Geometry: final body of the model. Coordinates: model frame, mm. Face numbers are marked on the shaded views. A direction names the side the tool comes from. Give positions to 0.01 mm unless a question says otherwise; leave off trailing zeros. Order: outer loops, then holes, each group sorted by start corner. A loop starts at its lowest first (then second) coordinate and runs counter-clockwise, first axis right, second up. Notation, with made-up numbers: (51, 2.25) - (87, 2.25) arc R8 cw to (87, 6.25) - close; hole circle Ø11 at (88, -9). An arc over 180 degrees is marked (long way). Put each result on its own line as item: value. Start each with the question number.
1. Section A-A on y = 0.75. Return the cut outline in (x, z).
2. Section B-B on x = -12.7. Return the cut outline in (y, z), plus the area to 4 significant figures.
3. Ray query, line 1 along X through (y, z) = (5, 1.25); line 2 along Y through (x, z) = (12.7, 0.15); line 3 along X through (y, z) = (-4, 1.65). Return the intervals inside material, ascending. Write a range as from..to.
4. Section C-C on x = 21.5. Return the cut outline in (y, z).
5. Set-up query: the marked faces 1 and 2. Return all of +Z, -Z, +X, -X, +Y, -Y with unobstructed straight access to the full face (end or side cutting, diameter ignored); none if empty.
6. First-contact query: P1, Ø1.5, axis at y = 7.5, z = 1, coming from the +X side; P2, Ø0.8, axis at y = 4.5, z = 1, coming from the +X side; P3, Ø0.8, axis at x = 3.5, y = -10, coming from the -Z side. Flat tips, straight axial feed; report the tip coordinate or a pass-through.
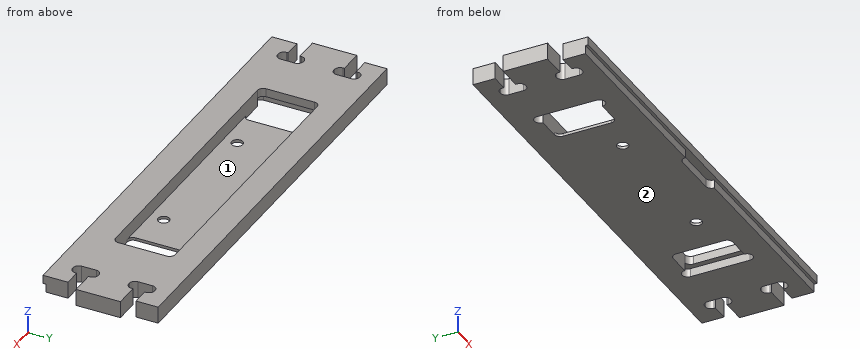
from build123d import *

# Parameters (mm, degrees)
SKETCH1_W                          = 1.3
SKETCH1_H                          = 7.9
BASE_SHAPE_DEPTH                   = 3
SKETCH4_W                          = 79
SKETCH4_H                          = 1.5
FLOOR_LIP_DEPTH                    = 0.5
NAIL_CUTOUT_DEPTH                  = 1.5
MILL_FILLETS_R                     = 1
LED_STRIP_POCKET_DEPTH             = 2.5
LED_STRIP_CUTS_REACH               = 2.5
SKETCH9_R                          = 1
LED_STRIP_CUT_FILLETS_R            = 1
LED_PCB_PADS_CLEARANCE_SLOTS_DEPTH = 1.5


with BuildPart() as part:
    # Sketch1 → Base shape (new body)
    with BuildSketch(Plane.XY):
        Polygon((39.5, 10), (-39.5, 10), (-39.5, 6.05), (-36.5, 6.05), (-36.5, 7.3), (-34.3, 7.3), (-34.3, 2.7), (-36.5, 2.7), (-36.5, 3.95), (-39.5, 3.95), (-39.5, -3.95), (-36.5, -3.95), (-36.5, -2.7), (-34.3, -2.7), (-34.3, -7.3), (-36.5, -7.3), (-36.5, -6.05), (-39.5, -6.05), (-39.5, -10), (39.5, -10), (39.5, -6.05), (36.5, -6.05), (36.5, -7.3), (34.3, -7.3), (34.3, -2.7), (36.5, -2.7), (36.5, -3.95), (39.5, -3.95), (39.5, 3.95), (36.5, 3.95), (36.5, 2.7), (34.3, 2.7), (34.3, 7.3), (36.5, 7.3), (36.5, 6.05), (39.5, 6.05), align=None)
        with Locations((-40.15, 0)):
            Rectangle(SKETCH1_W, SKETCH1_H)
        with Locations((40.15, 0)):
            Rectangle(SKETCH1_W, SKETCH1_H)
    extrude(amount=BASE_SHAPE_DEPTH)

    # Sketch4 → Floor lip (add)
    with BuildSketch(Plane.XZ.offset(10)):
        with Locations((0, 2.25)):
            Rectangle(SKETCH4_W, SKETCH4_H)
    extrude(amount=FLOOR_LIP_DEPTH)

    # Sketch6 → Nail cutout (cut)
    with BuildSketch(Plane(origin=(0, 0, 0), x_dir=(-1, 0, 0), z_dir=(0, 0, -1))):
        with BuildLine():
            Line((-4, -9), (4, -9))
            ThreePointArc((4, -9), (5, -10), (4, -11))
            Line((4, -11), (-4, -11))
            ThreePointArc((-4, -11), (-5, -10), (-4, -9))
        make_face()
    extrude(amount=-NAIL_CUTOUT_DEPTH, mode=Mode.SUBTRACT)

    # Mill fillets
    mill_fillets_edges = [part.edges().sort_by_distance(p)[0] for p in [
        (36.5, -2.7, 1.5),
        (34.3, -2.7, 1.5),
        (34.3, -7.3, 1.5),
        (36.5, -7.3, 1.5),
        (-36.5, -7.3, 1.5),
        (-34.3, -7.3, 1.5),
        (-34.3, -2.7, 1.5),
        (-36.5, -2.7, 1.5),
        (-36.5, 2.7, 1.5),
        (-34.3, 2.7, 1.5),
        (-34.3, 7.3, 1.5),
        (-36.5, 7.3, 1.5),
        (36.5, 7.3, 1.5),
        (34.3, 7.3, 1.5),
        (34.3, 2.7, 1.5),
        (36.5, 2.7, 1.5),
    ]]
    fillet(mill_fillets_edges, radius=MILL_FILLETS_R)

    # Sketch8 → Led strip pocket (cut)
    with BuildSketch(Plane.XY.offset(3)):
        with BuildLine():
            Line((-24.5, 5.3), (24.5, 5.3))
            ThreePointArc((24.5, 5.3), (25.207106781, 5.007106781), (25.5, 4.3))
            Line((25.5, 4.3), (25.5, -4.3))
            ThreePointArc((25.5, -4.3), (25.207106781, -5.007106781), (24.5, -5.3))
            Line((24.5, -5.3), (-24.5, -5.3))
            ThreePointArc((-24.5, -5.3), (-25.207106781, -5.007106781), (-25.5, -4.3))
            Line((-25.5, -4.3), (-25.5, 4.3))
            ThreePointArc((-25.5, 4.3), (-25.207106781, 5.007106781), (-24.5, 5.3))
        make_face()
    extrude(amount=-LED_STRIP_POCKET_DEPTH, mode=Mode.SUBTRACT)

    # Sketch9 → Led strip cuts (cut, up to next)
    with BuildSketch(Plane.XY.offset(0.5), mode=Mode.PRIVATE) as led_strip_cuts_sk1:
        with BuildLine():
            Line((-19.5, -5.3), (-19.5, 5.3))
            Line((-19.5, 5.3), (-24.5, 5.3))
            ThreePointArc((-24.5, 5.3), (-25.207106781, 5.007106781), (-25.5, 4.3))
            Line((-25.5, 4.3), (-25.5, -4.3))
            ThreePointArc((-25.5, -4.3), (-25.207106781, -5.007106781), (-24.5, -5.3))
            Line((-24.5, -5.3), (-19.5, -5.3))
        make_face()
    led_strip_cuts_tool1 = extrude(led_strip_cuts_sk1.sketch, amount=-LED_STRIP_CUTS_REACH, mode=Mode.PRIVATE) & part.part
    add(led_strip_cuts_tool1.solids().sort_by_distance((-22.481135, 0, 0.5))[0], mode=Mode.SUBTRACT)
    # Sketch9 → Led strip cuts (cut, up to next)
    with BuildSketch(Plane.XY.offset(0.5), mode=Mode.PRIVATE) as led_strip_cuts_sk2:
        with BuildLine():
            Line((24.5, 5.3), (19.5, 5.3))
            Line((19.5, 5.3), (19.5, -5.3))
            Line((19.5, -5.3), (24.5, -5.3))
            ThreePointArc((24.5, -5.3), (25.207106781, -5.007106781), (25.5, -4.3))
            Line((25.5, -4.3), (25.5, 4.3))
            ThreePointArc((25.5, 4.3), (25.207106781, 5.007106781), (24.5, 5.3))
        make_face()
    led_strip_cuts_tool2 = extrude(led_strip_cuts_sk2.sketch, amount=-LED_STRIP_CUTS_REACH, mode=Mode.PRIVATE) & part.part
    add(led_strip_cuts_tool2.solids().sort_by_distance((22.481135, 0, 0.5))[0], mode=Mode.SUBTRACT)
    # Sketch9 → Led strip cuts (cut, up to next)
    with BuildSketch(Plane.XY.offset(0.5), mode=Mode.PRIVATE) as led_strip_cuts_sk3:
        with Locations((-12.7, -2.828)):
            Circle(SKETCH9_R)
    led_strip_cuts_tool3 = extrude(led_strip_cuts_sk3.sketch, amount=-LED_STRIP_CUTS_REACH, mode=Mode.PRIVATE) & part.part
    add(led_strip_cuts_tool3.solids().sort_by_distance((-12.7, -2.828, 0.5))[0], mode=Mode.SUBTRACT)
    # Sketch9 → Led strip cuts (cut, up to next)
    with BuildSketch(Plane.XY.offset(0.5), mode=Mode.PRIVATE) as led_strip_cuts_sk4:
        with Locations((12.7, -2.828)):
            Circle(SKETCH9_R)
    led_strip_cuts_tool4 = extrude(led_strip_cuts_sk4.sketch, amount=-LED_STRIP_CUTS_REACH, mode=Mode.PRIVATE) & part.part
    add(led_strip_cuts_tool4.solids().sort_by_distance((12.7, -2.828, 0.5))[0], mode=Mode.SUBTRACT)

    # Led strip cut fillets
    led_strip_cut_fillets_edges = [part.edges().sort_by_distance(p)[0] for p in [
        (-19.5, 5.3, 0.25),
        (-19.5, -5.3, 0.25),
        (19.5, 5.3, 0.25),
        (19.5, -5.3, 0.25),
    ]]
    fillet(led_strip_cut_fillets_edges, radius=LED_STRIP_CUT_FILLETS_R)

    # Sketch23 → LED PCB pads clearance slots (cut)
    with BuildSketch(Plane(origin=(0, 0, 0), x_dir=(-1, 0, 0), z_dir=(0, 0, -1))):
        with BuildLine():
            Line((-26.5, -5.3), (-26.5, 5.3))
            ThreePointArc((-26.5, 5.3), (-25.5, 6.3), (-24.5, 5.3))
            Line((-24.5, 5.3), (-24.5, -5.3))
            ThreePointArc((-24.5, -5.3), (-25.5, -6.3), (-26.5, -5.3))
        make_face()
        with BuildLine():
            Line((26.5, -5.3), (26.5, 5.3))
            ThreePointArc((26.5, 5.3), (25.5, 6.3), (24.5, 5.3))
            Line((24.5, 5.3), (24.5, -5.3))
            ThreePointArc((24.5, -5.3), (25.5, -6.3), (26.5, -5.3))
        make_face()
    extrude(amount=-LED_PCB_PADS_CLEARANCE_SLOTS_DEPTH, mode=Mode.SUBTRACT)


solid = part.part
Resolved:
1. outline: (-40.8, 0) - (-26.5, 0) - (-26.5, 1.5) - (-25.5, 1.5) - (-25.5, 3) - (-40.8, 3) - close; (-19.5, 0) - (19.5, 0) - (19.5, 0.5) - (-19.5, 0.5) - close; (25.5, 1.5) - (26.5, 1.5) - (26.5, 0) - (40.8, 0) - (40.8, 3) - (25.5, 3) - close
2. outline: (-10.5, 1.5) - (-10, 1.5) - (-10, 0) - (-3.83, 0) - (-3.83, 0.5) - (-5.3, 0.5) - (-5.3, 3) - (-10.5, 3) - close; (-1.83, 0) - (10, 0) - (10, 3) - (5.3, 3) - (5.3, 0.5) - (-1.83, 0.5) - close
2. area: 33.25 mm^2
3. line 1: -34.3..-26.5, 26.5..34.3
3. line 2: -10..-3.83, -1.83..10
3. line 3: -34.3..-25.5, 25.5..34.3
4. outline: (-10.5, 1.5) - (-10, 1.5) - (-10, 0) - (-5.3, 0) - (-5.3, 3) - (-10.5, 3) - close; (5.3, 0) - (10, 0) - (10, 3) - (5.3, 3) - close
5. face 1: +Z
5. face 2: -Z, +X, -X, +Y, -Y
6. P1: x = 39.5
6. P2: x = 34.3
6. P3: z = 1.5
